```python
from build123d import *

# Parameters (mm, degrees)
SKETCH1_W                                          = 101.6
SKETCH1_H                                          = 127
BOSS_EXTRUDE1_DEPTH                                = 3.175
SKETCH2_W                                          = 4.7625
SKETCH2_H                                          = 2.38125
BOSS_EXTRUDE2_DEPTH                                = 1.190625
FILLET1_R                                          = 2.54
BOSS_EXTRUDE3_DEPTH                                = 5.55625
CBORE_FOR_M2_5_HEX_HEAD_MACHINE_SCREW1_D           = 2.7
CBORE_FOR_M2_5_HEX_HEAD_MACHINE_SCREW1_CBORE_D     = 7.28
CBORE_FOR_M2_5_HEX_HEAD_MACHINE_SCREW1_CBORE_DEPTH = 2.1
SKETCH8_R                                          = 6.35
CUT_EXTRUDE1_DEPTH                                 = 148.63326429


with BuildPart() as part:
    # Sketch1 → Boss-Extrude1 (new body)
    with BuildSketch(Plane(origin=(0, 0, 0), x_dir=(1, 0, 0), z_dir=(0, 1, 0))):
        with Locations((0, 63.5)):
            Rectangle(SKETCH1_W, SKETCH1_H)
    extrude(amount=BOSS_EXTRUDE1_DEPTH)

    # Sketch2 → Boss-Extrude2 (add)
    with BuildSketch(Plane.XZ):
        with Locations((-22.225, 1.190625)):
            Rectangle(SKETCH2_W, SKETCH2_H)
        with Locations((22.225, 1.190625)):
            Rectangle(SKETCH2_W, SKETCH2_H)
    extrude(amount=-BOSS_EXTRUDE2_DEPTH)

    # Fillet1
    fillet1_edges = [part.edges().sort_by_distance(p)[0] for p in [
        (50.8, 1.5875, 0),
        (-50.8, 1.5875, 0),
        (-50.8, 1.5875, -127),
        (50.8, 1.5875, -127),
    ]]
    fillet(fillet1_edges, radius=FILLET1_R)

    # Sketch4 → Boss-Extrude3 (add, symmetric)
    with BuildSketch(Plane(origin=(0, 0, 0), x_dir=(0, 0, -1), z_dir=(1, 0, 0))):
        with BuildLine():
            Line((120.65, 0), (126.111050725, -5.461050725))
            ThreePointArc((126.111050725, -5.461050725), (128.301155995, -6.024193053), (129.850888229, -4.377371758))
            Line((129.850888229, -4.377371758), (130.175, -2.936875))
            Line((130.175, -2.936875), (128.5875, -2.936875))
            Line((128.5875, -2.936875), (128.5875, 6.588125))
            Line((128.5875, 6.588125), (138.1125, 6.588125))
            Line((138.1125, 6.588125), (138.1125, 4.048125))
            Line((138.1125, 4.048125), (131.1275, 4.048125))
            Line((131.1275, 4.048125), (131.1275, -0.396875))
            Line((131.1275, -0.396875), (133.35, -0.396875))
            Line((133.35, -0.396875), (132.32893701, -4.934932733))
            ThreePointArc((132.32893701, -4.934932733), (129.008082223, -8.463835508), (124.314999501, -7.25710195))
            Line((124.314999501, -7.25710195), (117.057897552, 0))
            Line((117.057897552, 0), (120.65, 0))
        make_face()
    extrude(amount=BOSS_EXTRUDE3_DEPTH, both=True)

    # CBORE for M2.5 Hex Head Machine Screw1 (through all)
    with Locations(Plane(origin=(0, 0, 0), x_dir=(-1, 0, 0), z_dir=(0, -1, 0))):
        with Locations((20, 36.435847812), (28, 106.435847812), (-20, 36.435847812), (-28, 106.435847812)):
            CounterBoreHole(CBORE_FOR_M2_5_HEX_HEAD_MACHINE_SCREW1_D / 2, CBORE_FOR_M2_5_HEX_HEAD_MACHINE_SCREW1_CBORE_D / 2, CBORE_FOR_M2_5_HEX_HEAD_MACHINE_SCREW1_CBORE_DEPTH)

    # Sketch8 → Cut-Extrude1 (cut, through all)
    with BuildSketch(Plane(origin=(0, 3.175, 0), x_dir=(1, 0, 0), z_dir=(0, 1, 0))):
        with Locations(Location((0, 50.8, 0), (0, 0, 270))):
            Circle(SKETCH8_R)
    extrude(amount=-CUT_EXTRUDE1_DEPTH, mode=Mode.SUBTRACT)


solid = part.part
```
Verification items for the finished model (mm, model axes). A direction names the side the tool comes from. Coordinates: 2 decimals unless noted, no trailing zeros. Order: outer loops, then holes, each group sorted by start corner. A loop starts at its lowest first (then second) coordinate and runs counter-clockwise, first axis right, second up. Notation, with made-up numbers: (48, -20) - (102, -20) arc R16 ccw to (102, -2) - close; hole circle Ø8 at (-33, 56.25). An arc over 180 degrees is marked (long way). Return JSON: item names as keys, results as strings.
(1) Thickness scan on line 1 along Z through (x, y) = (-28, 2.95); line 2 along Z through (x, y) = (-20, 0.95); line 3 along Y through (x, z) = (-34, -121.5) (3 decimals). Record the ranges inside material, lowest first.
Filled sheet:
{"line 1": "z = -127 to -107.79, -105.09 to 0", "line 2": "z = -127 to -40.08, -32.8 to 2.38", "line 3": "y = 0 to 3.175"}
(2) Access from +Z, -Z, +X, -X, +Y, -Y to the whole of each face (thin tool, end or side, straight path). Record for faces 5 (the cylindrical face through (0.078, -8.444, -129.076)), 6 (the flat face through (-27.9, 2.1, -104.9)).
Filled sheet:
{"face 5": "+X, -X, -Y", "face 6": "-Y"}
(3) Section check A-A, the plane z = -50.8. Record the cut outline in (x, y) (3 decimals).
Filled sheet:
{"outline": "(-50.8, 0) - (-6.35, 0) - (-6.35, 3.175) - (-50.8, 3.175) - close; (6.35, 0) - (50.8, 0) - (50.8, 3.175) - (6.35, 3.175) - close"}
(4) Go/stop test with flat-tipped pins: pin 1 (1.5 mm diameter, centred on x = 28.5, z = -65.5, fed in from -Y); pin 2 (1 mm diameter, centred on y = 0.5, z = 1.5, fed in from +X); pin 3 (2 mm diameter, centred on x = 39.5, y = 2, fed in from +Z); pin 4 (5 mm diameter, centred on x = 33.5, y = -4.5, fed in from -Z). Record where each tip stops, or that it passes through.
Filled sheet:
{"pin 1": "stops at y = 0", "pin 2": "stops at x = 24.61", "pin 3": "stops at z = 0", "pin 4": "passes through"}
(5) Mould release check, pull along Y, two halves, no side actions. Record for faces 1 (the cylindrical face through (0.078, -6.033, -128.269)), 2 (the flat face through (0, 2, -131.128)), 3 (the flat face through (0, 2, -128.588)), 4 (the flat face through (28.1, 2.1, -104.9)): pulls with the +Y half, pulls with the -Y half, needs draft (parallel to the pull), parting line crosses it, or undercut.
Filled sheet:
{"face 1": "undercut", "face 2": "undercut", "face 3": "needs draft", "face 4": "pulls with the -Y half"}
(6) Section check C-C, the plane z = -75. Record the cut outline in (x, y) (3 decimals).
Filled sheet:
{"outline": "(-50.8, 0) - (50.8, 0) - (50.8, 3.175) - (-50.8, 3.175) - close"}
